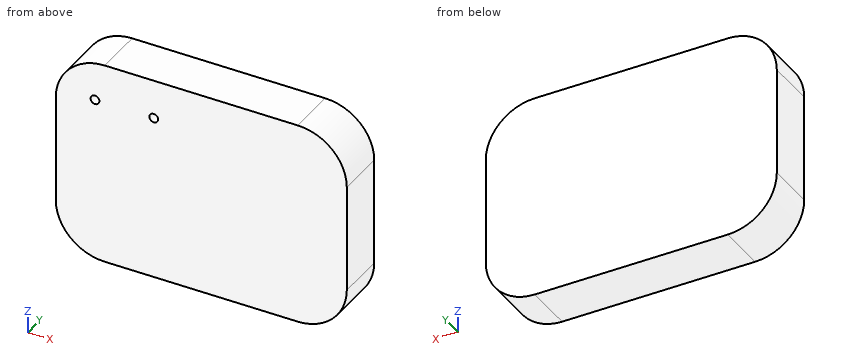
```python
from build123d import *

# Parameters (mm, degrees)
F2_DEPTH = 9
F3_R     = 4.5
F4_DEPTH = 25
F6_DEPTH = 25
F7_DEPTH = 25
F8_R     = 4.5
F9_DEPTH = 25


with BuildPart() as f2:
    # F0 (on Front) → F2 (new body)
    with BuildSketch(Plane.XZ):
        with BuildLine():
            Line((89.0472261183, 101.7465810478), (-107.9527738817, 101.7465810478))
            ThreePointArc((-107.9527738817, 101.7465810478), (-143.308112941, 87.1019201071), (-157.9527738817, 51.7465810478))
            Line((-157.9527738817, 51.7465810478), (-157.9527738817, -58.2534189522))
            ThreePointArc((-157.9527738817, -58.2534189522), (-143.308112941, -93.6087580116), (-107.9527738817, -108.2534189522))
            Line((-107.9527738817, -108.2534189522), (89.0472261183, -108.2534189522))
            ThreePointArc((89.0472261183, -108.2534189522), (124.4025651777, -93.6087580116), (139.0472261183, -58.2534189522))
            Line((139.0472261183, -58.2534189522), (139.0472261183, 51.7465810478))
            ThreePointArc((139.0472261183, 51.7465810478), (124.4025651777, 87.1019201071), (89.0472261183, 101.7465810478))
        make_face()
    extrude(amount=F2_DEPTH)

    # F3 (on face) → F4 (join)
    with BuildSketch(Plane.XZ.offset(9)):
        with Locations((-117.9527738817, 61.7465810478)):
            Circle(F3_R)
        with Locations((-57.9527738817, 61.7465810478)):
            Circle(F3_R)
    extrude(amount=F4_DEPTH)

    # F5 (on face) → F6 (cut)
    with BuildSketch(Plane.XZ.offset(9)):
        with BuildLine():
            Line((138.772751035, 56.9784231484), (61.5566782653, 56.9784231484))
            Line((61.5566782653, 56.9784231484), (61.5566782653, 26.1754468083))
            Line((61.5566782653, 26.1754468083), (139.0472261183, 26.1754468083))
            Line((139.0472261183, 26.1754468083), (139.0472261183, 51.7465810478))
            ThreePointArc((139.0472261183, 51.7465810478), (138.9785601974, 54.3660995311), (138.772751035, 56.9784231484))
        make_face()
    extrude(amount=-F6_DEPTH, mode=Mode.SUBTRACT)

    # F1 (on face) → F7 (join)
    with BuildSketch(Plane.XZ):
        with BuildLine():
            ThreePointArc((139.0472261183, 51.7465810478), (124.4025651777, 87.1019201071), (89.0472261183, 101.7465810478))
            Line((89.0472261183, 101.7465810478), (-107.9527738817, 101.7465810478))
            ThreePointArc((-107.9527738817, 101.7465810478), (-143.308112941, 87.1019201071), (-157.9527738817, 51.7465810478))
            Line((-157.9527738817, 51.7465810478), (-157.9527738817, -58.2534189522))
            ThreePointArc((-157.9527738817, -58.2534189522), (-143.308112941, -93.6087580116), (-107.9527738817, -108.2534189522))
            Line((-107.9527738817, -108.2534189522), (89.0472261183, -108.2534189522))
            ThreePointArc((89.0472261183, -108.2534189522), (124.4025651777, -93.6087580116), (139.0472261183, -58.2534189522))
            Line((139.0472261183, -58.2534189522), (139.0472261183, 51.7465810478))
        make_face()
    extrude(amount=F7_DEPTH)

    # F8 (on face) → F9 (join)
    with BuildSketch(Plane.XZ.offset(25)):
        with BuildLine():
            Line((-107.9527738817, -108.2534189522), (89.0472261183, -108.2534189522))
            ThreePointArc((89.0472261183, -108.2534189522), (124.4025651777, -93.6087580116), (139.0472261183, -58.2534189522))
            Line((139.0472261183, -58.2534189522), (139.0472261183, 51.7465810478))
            ThreePointArc((139.0472261183, 51.7465810478), (124.4025651777, 87.1019201071), (89.0472261183, 101.7465810478))
            Line((89.0472261183, 101.7465810478), (-107.9527738817, 101.7465810478))
            ThreePointArc((-107.9527738817, 101.7465810478), (-143.308112941, 87.1019201071), (-157.9527738817, 51.7465810478))
            Line((-157.9527738817, 51.7465810478), (-157.9527738817, -58.2534189522))
            ThreePointArc((-157.9527738817, -58.2534189522), (-143.308112941, -93.6087580116), (-107.9527738817, -108.2534189522))
        make_face()
        with Locations((-117.9527738817, 61.7465810478)):
            Circle(F8_R, mode=Mode.SUBTRACT)
        with Locations((-57.9527738817, 61.7465810478)):
            Circle(F8_R, mode=Mode.SUBTRACT)
    extrude(amount=F9_DEPTH)


solid = f2.part
```
Can you work these out from the model? Positions are in its coordinate system, mm. Coordinates: 2 decimals unless noted, no trailing zeros. Loops run counter-clockwise (first coordinate to the right, second up) from the corner with the lowest first, then second, coordinate; pieces in that order, holes last. Notation, with made-up numbers: (68.5, 44) -> (93.5, 44) arc R35 cw to (93.5, 82) -> close; hole circle Ø4 at (-22.75, 52.5). An arc over 180 degrees is marked (long way). Answer as a JSON object with one key per item and string values.
1) If I drill on line 1 (X direction, y = -17, z = -91.5); line 2 (X direction, y = -10.5, z = 67.5); line 3 (Z direction, x = 116, y = -30), over which ranges is the centre line in solid material (lowest first)?
Results:
{"line 1": "x = -145.3 to 126.39", "line 2": "x = -155.41 to 136.5", "line 3": "z = -100.37 to 93.86"}
2) For P1, Ø10, axis at x = -56.5, z = 63.5, coming from the -Y side; P2, Ø3, axis at x = 91, y = -16, coming from the -Z side; P3, Ø2, axis at y = -39, z = -71, coming from the +X side; P4, Ø4, axis at y = -18, z = -76.5, coming from the +X side, each with a flat end and sliding along its axis, tell me the tip position at first contact or that it passes through.
Results:
{"P1": "stops at y = -50", "P2": "stops at z = -108.25", "P3": "stops at x = 137.65", "P4": "stops at x = 136.33"}
3) Imagine slicing it at D-D (x = -133). Please give me the cut outline in (y, z), then the cut area to 3 significant figures.
Results:
{"outline": "(-50, -101.53) -> (0, -101.53) -> (0, 95.02) -> (-50, 95.02) -> close", "area": "9,830 mm^2"}
4) Imagine slicing it at A-A (y = -44). Please give me the cut outline in (x, z).
Results:
{"outline": "(-157.95, -58.25) arc R50 ccw to (-107.95, -108.25) -> (89.05, -108.25) arc R50 ccw to (139.05, -58.25) -> (139.05, 51.75) arc R50 ccw to (89.05, 101.75) -> (-107.95, 101.75) arc R50 ccw to (-157.95, 51.75) -> close; hole circle Ø9 at (-117.95, 61.75); hole circle Ø9 at (-57.95, 61.75)"}
5) Imagine slicing it at C-C (z = 70). Please give me the cut outline in (x, y), then the cut area to 3 significant figures.
Results:
{"outline": "(-154.5, -50) -> (135.6, -50) -> (135.6, 0) -> (-154.5, 0) -> close", "area": "14,500 mm^2"}
6) Imagine slicing it at B-B (y = -9). Please give me the cut outline in (x, z).
Results:
{"outline": "(-157.95, -58.25) arc R50 ccw to (-107.95, -108.25) -> (89.05, -108.25) arc R50 ccw to (139.05, -58.25) -> (139.05, 51.75) arc R50 ccw to (89.05, 101.75) -> (-107.95, 101.75) arc R50 ccw to (-157.95, 51.75) -> close"}
